Answer from the drawing. Dimensions are ordinates in mm from the lowest x, y and z of the part. A direction names the side the tool comes from. Round coordinates to 2 decimals unless told otherwise and drop trailing zeros. Order: outer loops, then holes, each group sorted by start corner. A loop starts at its lowest first (then second) coordinate and runs counter-clockwise, first axis right, second up.
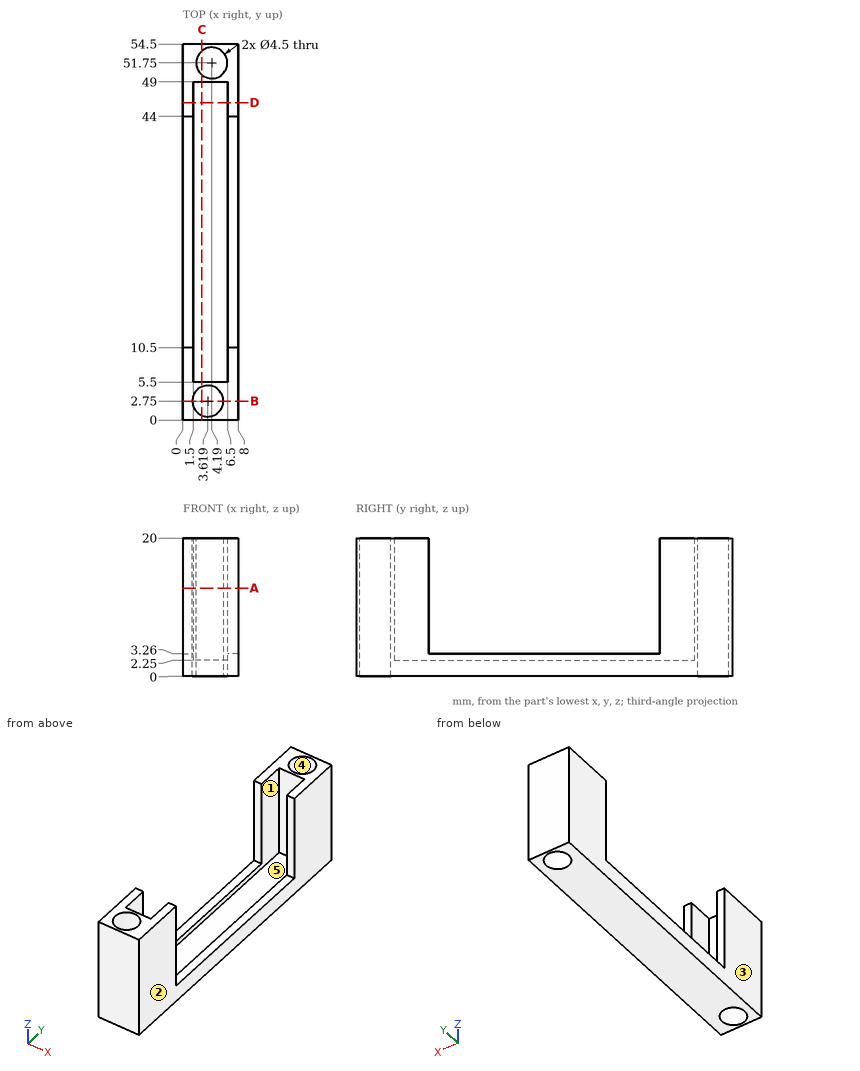
Q1. A cutting plane is placed at A-A, the plane z = 12.75. Give the vertices of the cut face in (x, y).
Outcome:
outline: (0, 0) - (8, 0) - (8, 10.5) - (6.5, 10.5) - (6.5, 5.5) - (1.5, 5.5) - (1.5, 10.5) - (0, 10.5) - close; (0, 44) - (1.5, 44) - (1.5, 49) - (6.5, 49) - (6.5, 44) - (8, 44) - (8, 54.5) - (0, 54.5) - close; hole circle Ø4.5 at (3.62, 2.75); hole circle Ø4.5 at (4.19, 51.75)
Q2. For a pull along X with two mould halves and no side action, classify the marked faces 1, 2 and 3 as released by +X, released by -X, zero draft, split by the parting line, or undercut.
Outcome:
face 1: undercut
face 2: released by +X
face 3: released by -X
Q3. A flat-ended cylindrical pin translates along its axis: pin 1 (1.6 mm diameter, centred on x = 7.5, y = 23.5, fed in from +Z). Find the tip coordinate at first contact, or state that the pin passes through.
Outcome:
pin 1: stops at z = 3.26
Q4. A cutting plane is placed at B-B, the plane y = 2.75. Give the vertices of the cut face in (x, z).
Outcome:
outline: (0, 0) - (1.37, 0) - (1.37, 20) - (0, 20) - close; (5.87, 0) - (8, 0) - (8, 20) - (5.87, 20) - close
Q5. Straight lines are drawn through the part: probe 1 along Y at (x, z) = (3.5, 11.5); probe 2 along Y at (x, z) = (2.5, 19) (1 decimal); probe 3 along X at (y, z) = (28, 3). For each, find the intervals that lie inside material, in ascending order.
Outcome:
probe 1: y = 0 to 0.5, 5 to 5.5, 49 to 49.61, 53.89 to 54.5
probe 2: y = 0 to 0.8, 4.7 to 5.5, 49 to 50.3, 53.2 to 54.5
probe 3: x = 0 to 1.5, 6.5 to 8
Q6. For the marked faces 4 and 5, determine the directions among +Z, -Z, +X, -X, +Y, -Y from which every point of the face is accessible in a straight line to the end or side of a thin tool.
Outcome:
face 4: +Z, -Z
face 5: +Z
Q7. A cutting plane is placed at D-D, the plane y = 46. Give the vertices of the cut face in (x, z).
Outcome:
outline: (0, 0) - (8, 0) - (8, 20) - (6.5, 20) - (6.5, 2.25) - (1.5, 2.25) - (1.5, 20) - (0, 20) - close
Q8. A cutting plane is placed at C-C, the plane x = 2.75. Give the number of separate pieces and of enclosed holes in the cut face, plus the area to 3 significant figures.
Outcome:
separate pieces: 3
enclosed holes: 0
area: 166 mm2
